Geometry: final body of the model. Coordinates: model frame, mm. Face numbers are marked on the shaded views. Give positions to 0.01 mm unless a question says otherwise; leave off trailing zeros. Write each loop counter-clockwise with the first axis right and the second up, starting at its lowest first coordinate (ties: lowest second). Pieces come first, ordered by that corner, then holes. Notation, with made-up numbers: M -21,-35 L 0,-35 A30 cw 0,1 Z; hole C 84,-26 d2. An arc over 180 degrees is marked long. One line per question, with ' | ' between items.
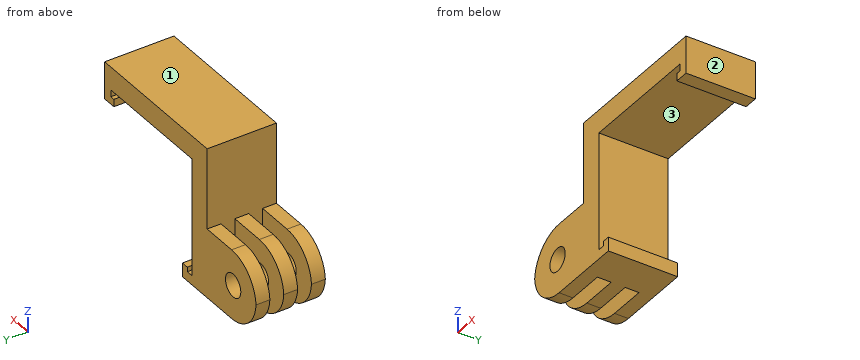
from build123d import *

# Parameters (mm, degrees)
F1_DEPTH    = 15
F2_W        = 3
F2_H        = 15
F3_DEPTH    = 16
F5_DEPTH    = 25
F6_T1_DEPTH = 43
F6_T3_DEPTH = 43
F6_T5_DEPTH = 43


# Not quite as in the source:
# - a fillet or chamfer that OpenCascade refuses, or shapes differently, is made with other operations: its cross-section is extruded or revolved along the edge and cut away or added


with BuildPart() as f1:
    # F0 (on Front) → F1 (new body)
    with BuildSketch(Plane.XZ):
        Polygon((0, -23.585311383), (0, 0), (25, 0), (26.5, 0), (26.5, -1.5), (25.5, -1.5), (25.5, -3.1), (28.5, -3.1), (28.5, 5), (25, 5), (-5, 5), (-5, -24), (-5, -25.5), (-5, -27.5), (0, -27.5), (3.1, -27.5), (3.1, -24.5), (1.5, -24.5), (1.5, -25.5), (0, -25.5), (0, -25.085311383), align=None)
    extrude(amount=F1_DEPTH)

    # F2 (on face) → F3 (join)
    with BuildSketch(Plane(origin=(-5, 0, 0), x_dir=(0, -1, 0), z_dir=(-1, 0, 0))):
        with Locations((1.5, -20)):
            Rectangle(F2_W, F2_H)
        with Locations((7.5, -20)):
            Rectangle(F2_W, F2_H)
        with Locations((13.5, -20)):
            Rectangle(F2_W, F2_H)
    extrude(amount=F3_DEPTH)

    # F4 (on face) → F5 (cut)
    with BuildSketch(Plane.XZ.offset(15)):
        with BuildLine():
            ThreePointArc((-16, -20), (-13.5, -22.5), (-11, -20))
            ThreePointArc((-11, -20), (-13.5, -17.5), (-16, -20))
        make_face()
    extrude(amount=-F5_DEPTH, mode=Mode.SUBTRACT)

    # F6: fillet of radius 8 on 5 edges, made by hand

    # F6_s2 → F6_t1 (cut)
    with BuildSketch(Plane.XZ.offset(-8)):
        with BuildLine():
            ThreePointArc((-21, -20.5), (-18.6568542495, -14.8431457505), (-13, -12.5))
            Line((-13, -12.5), (-21, -12.5))
            Line((-21, -12.5), (-21, -20.5))
        make_face()
    extrude(amount=F6_T1_DEPTH, mode=Mode.SUBTRACT)

    # F6_s4 → F6_t3 (cut)
    with BuildSketch(Plane.XZ.offset(-14)):
        with BuildLine():
            ThreePointArc((-21, -20.5), (-18.6568542495, -14.8431457505), (-13, -12.5))
            Line((-13, -12.5), (-21, -12.5))
            Line((-21, -12.5), (-21, -20.5))
        make_face()
        with BuildLine():
            ThreePointArc((-13, -27.5), (-18.6568542495, -25.1568542495), (-21, -19.5))
            Line((-21, -19.5), (-21, -27.5))
            Line((-21, -27.5), (-13, -27.5))
        make_face()
    extrude(amount=F6_T3_DEPTH, mode=Mode.SUBTRACT)

    # F6_s6 → F6_t5 (cut)
    with BuildSketch(Plane.XZ.offset(-20)):
        with BuildLine():
            ThreePointArc((-21, -20.5), (-18.6568542495, -14.8431457505), (-13, -12.5))
            Line((-13, -12.5), (-21, -12.5))
            Line((-21, -12.5), (-21, -20.5))
        make_face()
        with BuildLine():
            ThreePointArc((-13, -27.5), (-18.6568542495, -25.1568542495), (-21, -19.5))
            Line((-21, -19.5), (-21, -27.5))
            Line((-21, -27.5), (-13, -27.5))
        make_face()
    extrude(amount=F6_T5_DEPTH, mode=Mode.SUBTRACT)


solid = f1.part
(1) Draft query along X for the marked faces 1, 2 and 3. Return one class per face: released by +X, released by -X, zero draft, split by the parting line, or undercut.
Working result:
face 1: zero draft | face 2: released by +X | face 3: undercut
(2) First-contact query: P1, Ø2.5, axis at x = 27, y = -4.5, coming from the -Z side; P2, Ø5, axis at y = -7.5, z = -17, coming from the +X side; P3, Ø8, axis at y = -8, z = -21.5, coming from the +X side. Flat tips, straight axial feed; report the tip coordinate or a pass-through.
Working result:
P1: stops at z = -3.1 | P2: stops at x = 0 | P3: stops at x = 3.1
(3) Cut plane D-D, the plane x = -18. Return loops of the section in (y, z) (3 decimals), then the cut area to 3 significant figures.
Working result:
outline: M -15,-25.745 L -12,-25.745 L -12,-14.255 L -15,-14.255 Z; M -9,-25.745 L -6,-25.745 L -6,-14.255 L -9,-14.255 Z; M -3,-25.745 L 0,-25.745 L 0,-14.255 L -3,-14.255 Z | area: 103 mm^2
(4) Cut plane A-A, the plane z = -1. Return loops of the section in (x, y), then the cut area to 3 significant figures.
Working result:
outline: M -5,-15 L 0,-15 L 0,0 L -5,0 Z; M 26.5,-15 L 28.5,-15 L 28.5,0 L 26.5,0 Z | area: 105 mm^2
(5) Cut plane B-B, the plane x = 1. Return loops of the section in (y, z).
Working result:
outline: M -15,-27.5 L 0,-27.5 L 0,-25.5 L -15,-25.5 Z; M -15,0 L 0,0 L 0,5 L -15,5 Z
(6) Material intervals for L1, parallel to Y at x = -16, z = -13.5; L2, parallel to X at y = -6.5, z = -11.5; L3, parallel to X at y = -5.5, z = -3, sorted ascending. Write a range as [from, to].
Working result:
L1: y = [-15, -12], [-9, -6], [-3, 0] | L2: x = [-5, 0] | L3: x = [-5, 0], [25.5, 28.5]
(7) Cut plane C-C, the plane z = -21.5. Return loops of the section in (x, y), then the cut area to 3 significant figures.
Working result:
outline: M -20.75,-15 L -15.5,-15 L -15.5,-12 L -20.75,-12 Z; M -20.75,-9 L -15.5,-9 L -15.5,-6 L -20.75,-6 Z; M -20.75,-3 L -15.5,-3 L -15.5,0 L -20.75,0 Z; M -11.5,-15 L 0,-15 L 0,0 L -11.5,0 L -11.5,-3 L -5,-3 L -5,-6 L -11.5,-6 L -11.5,-9 L -5,-9 L -5,-12 L -11.5,-12 Z | area: 181 mm^2
